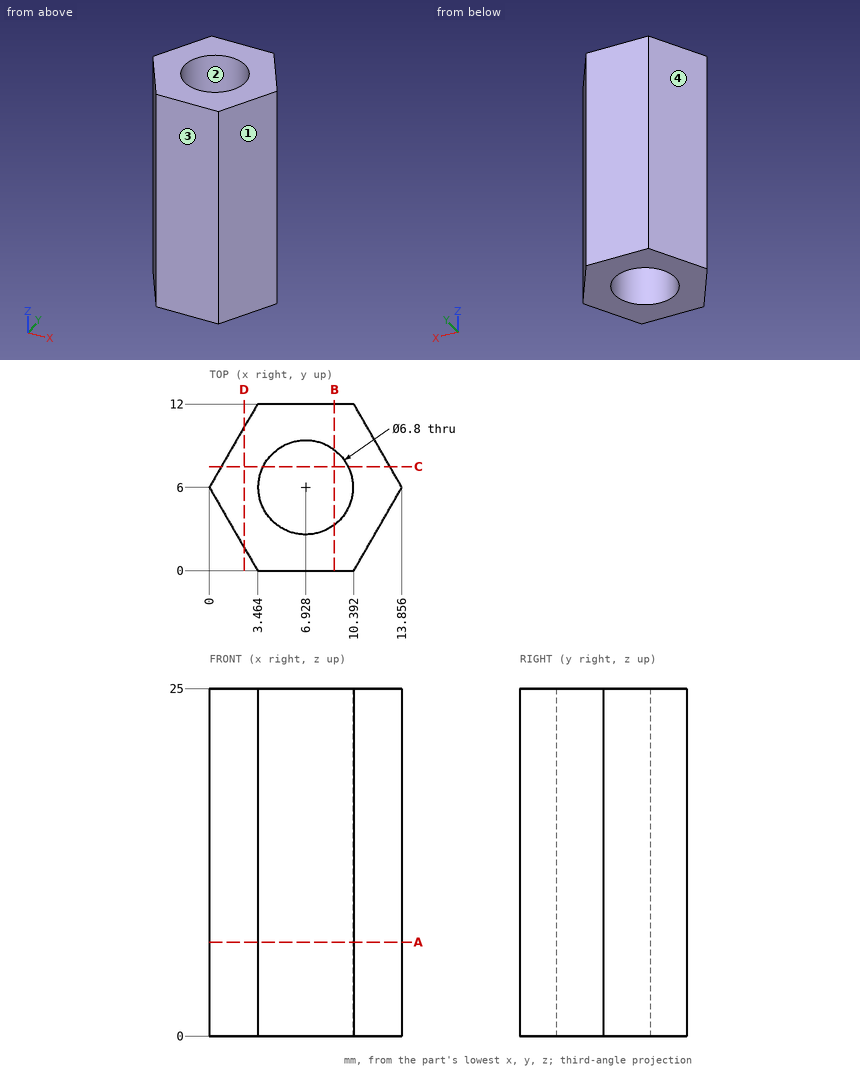
Study the drawing (mm; zero at the part's minimum x, y, z) and answer. Round coordinates to 2 decimals unless told otherwise and drop trailing zeros. Loops run counter-clockwise (first coordinate to the right, second up) from the corner with the lowest first, then second, coordinate; pieces in that order, holes last. Notation, with made-up numbers: (8.5, 86.5) -> (50.5, 86.5) arc R19 ccw to (50.5, 96.5) -> close; hole circle Ø3 at (-9.5, -24.75). An arc over 180 degrees is marked (long way). Write each question's results on one line, items separated by ' | '. Start each with the question number.
1. Given pin 1 Ø1.5 at (y, z) = (5, 15) entering from +X; pin 2 Ø4 at (y, z) = (1.5, 8) entering from -X; pin 3 Ø5.5 at (x, y) = (6.93, 6) entering from +Z, each flat-ended and moving along its own axis, determine where each tip first touches the part or whether it passes through.
2. For a pull along X with two mould halves and no side action, classify the marked faces 1, 2, 3 and 4 as +X half, -X half, draft (parallel to the pull), parting line (faces both ways), or undercut.
3. Section A-A (z = 6.75) is taken. Determine the outline of the cut face in (x, y).
4. Section B-B (x = 9) is taken. Determine the outline of the cut face in (y, z), plus the area to 3 significant figures.
5. Section D-D (x = 2.5) is taken. Determine the outline of the cut face in (y, z).
6. Find the intervals of material crossed by probe 1 along Y at (x, z) = (6.75, 12.75) (1 decimal); probe 2 along X at (y, z) = (4, 6.5) (1 decimal); probe 3 along Y at (x, z) = (4, 1.5) (1 decimal), in increasing order. Write a range as from..to.
7. Section C-C (y = 7.5) is taken. Determine the outline of the cut face in (x, z).
Evaluation:
1) pin 1: stops at x = 13.71 | pin 2: stops at x = 1.44 | pin 3: passes through
2) face 1: +X half | face 2: undercut | face 3: draft | face 4: -X half
3) outline: (0, 6) -> (3.46, 0) -> (10.39, 0) -> (13.86, 6) -> (10.39, 12) -> (3.46, 12) -> close; hole circle Ø6.8 at (6.93, 6)
4) outline: (0, 0) -> (3.3, 0) -> (3.3, 25) -> (0, 25) -> close; (8.7, 0) -> (12, 0) -> (12, 25) -> (8.7, 25) -> close | area: 165 mm2
5) outline: (1.67, 0) -> (10.33, 0) -> (10.33, 25) -> (1.67, 25) -> close
6) probe 1: y = 0..2.6, 9.4..12 | probe 2: x = 1.2..4.2, 9.7..12.7 | probe 3: y = 0..4.3, 7.7..12
7) outline: (0.87, 0) -> (3.88, 0) -> (3.88, 25) -> (0.87, 25) -> close; (9.98, 0) -> (12.99, 0) -> (12.99, 25) -> (9.98, 25) -> close
